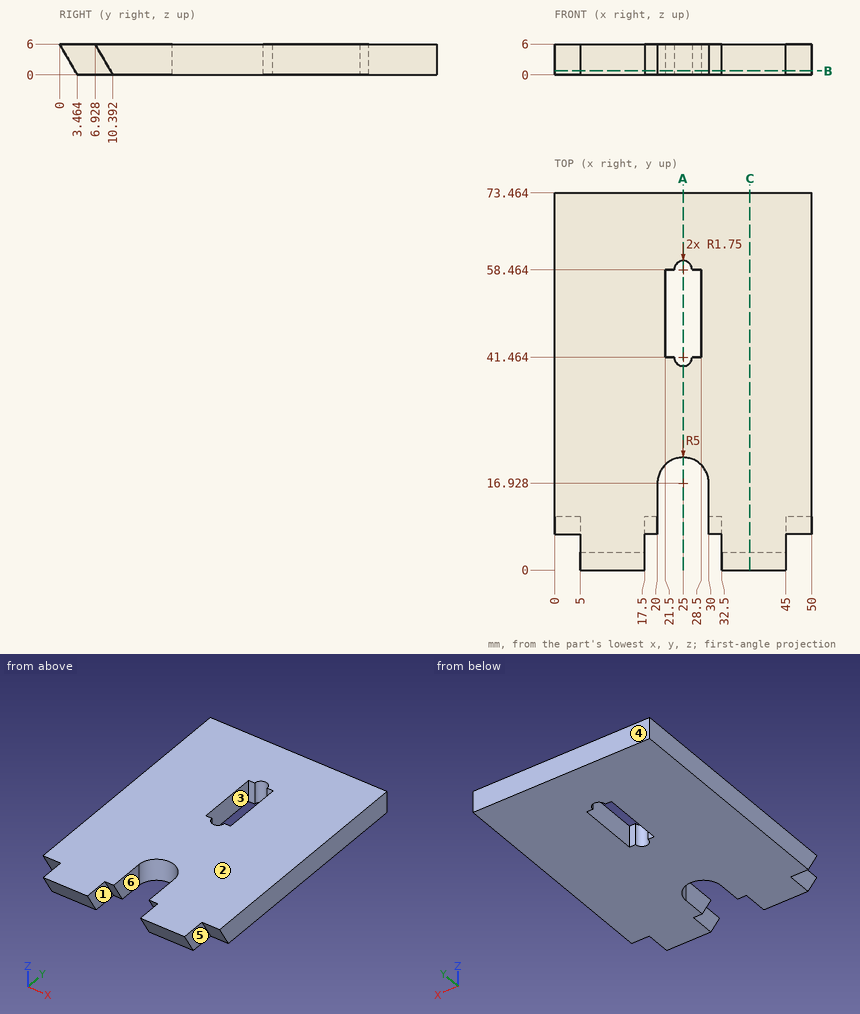
Input: dimensioned drawing with shaded views. Units: mm. Origin: part minimum x, y, z. A direction names the side the tool comes from. Coordinates: 2 decimals unless noted, no trailing zeros. Loops run counter-clockwise (first coordinate to the right, second up) from the corner with the lowest first, then second, coordinate; pieces in that order, holes last. Notation, with made-up numbers: M -13.75,10.5 L 3.25,10.5 A5 ccw 3.25,15.5 Z; hole C -22.5,21.5 d7. An arc over 180 degrees is marked long. Use a Markdown table: item, result. Add a question column.
Q1. Section query B-B, the plane z = 0.75. Return loops of the section in (x, y), and give its area (3 significant figures).
Q2. First-contact query: pin 1 (1 mm diameter, centred on y = 21.5, z = 1.5, fed in from -X); pin 2 (3 mm diameter, centred on y = 4.5, z = 2.5, fed in from +X); pin 3 (0.9 mm diameter, centred on x = 23, z = 4.5, fed in from -Y); pin 4 (1.9 mm diameter, centred on x = 28, z = 4, fed in from -Y) (1 decimal). Flat tips, straight axial feed; report the tip coordinate or a pass-through.
Q3. Section query A-A, the plane x = 25. Return loops of the section in (y, z), and give its area (3 significant figures).
Q4. Material intervals for L1, parallel to X at y = 11.5, z = 4.5; L2, parallel to X at y = 45, z = 3.75; L3, parallel to Y at x = 22.5, z = 4.5 (1 decimal), sorted ascending.
Q5. Draft query along X for the marked faces 4, 5 and 6. Return one class per face: pulls with the +X half, pulls with the -X half, needs draft (parallel to the pull), parting line crosses it, or undercut.
Q6. Section query C-C, the plane x = 38. Return loops of the section in (y, z).
Q7. Access query for the marked faces 1, 2 and 3. Directions: +Z, -Z, +X, -X, +Y, -Y. A direction counts if a zero-diameter tool reaches every point of the face in a straight line with its end or side. Return the directions, or none.
Result:
| question | item | result |
|---|---|---|
| 1 | outline | M 0,9.96 L 5,9.96 L 5,3.03 L 17.5,3.03 L 17.5,9.96 L 20,9.96 L 20,16.93 A5 cw 30,16.93 L 30,9.96 L 32.5,9.96 L 32.5,3.03 L 45,3.03 L 45,9.96 L 50,9.96 L 50,73.46 L 0,73.46 Z; hole M 21.5,41.46 L 23.25,41.46 A1.75 ccw 26.75,41.46 L 28.5,41.46 L 28.5,58.46 L 26.75,58.46 A1.75 ccw 23.25,58.46 L 21.5,58.46 Z |
| 1 | area | 3,110 mm2 |
| 2 | pin 1 | stops at x = 0 |
| 2 | pin 2 | stops at x = 45 |
| 2 | pin 3 | stops at y = 21.29 |
| 2 | pin 4 | stops at y = 20 |
| 3 | outline | M 21.93,0 L 39.71,0 L 39.71,6 L 21.93,6 Z; M 60.21,0 L 73.46,0 L 73.46,6 L 60.21,6 Z |
| 3 | area | 186 mm2 |
| 4 | L1 | x = 0 to 20, 30 to 50 |
| 4 | L2 | x = 0 to 21.5, 28.5 to 50 |
| 4 | L3 | y = 21.3 to 41.5, 58.5 to 73.5 |
| 5 | face 4 | needs draft |
| 5 | face 5 | pulls with the +X half |
| 5 | face 6 | undercut |
| 6 | outline | M 0,6 L 3.46,0 L 73.46,0 L 73.46,6 Z |
| 7 | face 1 | -Z, -Y |
| 7 | face 2 | +Z, +X, -X, +Y, -Y |
| 7 | face 3 | +Z, -Z |
